Answer from the drawing. Dimensions are ordinates in mm from the lowest x, y and z of the part. Coordinates: 2 decimals unless noted, no trailing zeros. Order: outer loops, then holes, each group sorted by start corner. A loop starts at its lowest first (then second) coordinate and runs counter-clockwise, first axis right, second up. Notation, with made-up numbers: (-1, -30.75) - (33, -30.75) arc R12 cw to (33, -10.75) - close; hole circle Ø11 at (40.25, 14.25). An arc over 180 degrees is marked (long way). Answer as a JSON object with one key per item and string values. Group by question number.
1) Find the intervals of material crossed by line 1 along X through (y, z) = (47.5, 5); line 2 along X through (y, z) = (156, 6.5), in increasing order.
2) Section C-C (y = 167) is taken. Give the vertices of the cut face in (x, z).
3) Section B-B (x = 47.5) is taken. Give the vertices of the cut face in (y, z).
4) Section A-A (z = 3) is taken. Give the vertices of the cut face in (x, y).
5) Each of these flat-tipped pins is pushed along its axis until it touches: P1, Ø4, axis at y = 99.5, z = 1.5, coming from the -X side; P2, Ø5, axis at x = 9, z = 2.5, coming from the -Y side; P3, Ø1, axis at y = 130.5, z = 7, coming from the +X side; P4, Ø1, axis at y = 42.5, z = 3, coming from the +X side. Where does it stop, or does it pass through?
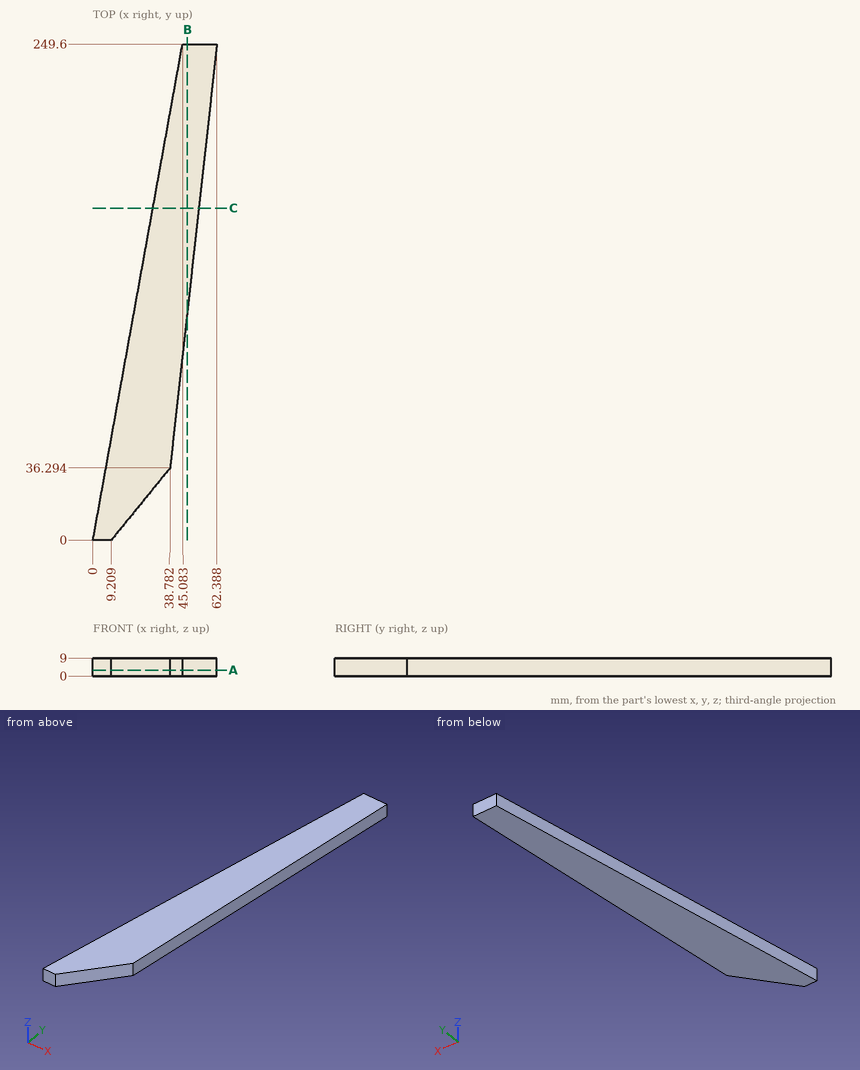
Report:
{
 "1": {"line 1": "x = 8.58 to 40.02", "line 2": "x = 28.18 to 52.03"},
 "2": {"outline": "(30.16, 0) - (53.25, 0) - (53.25, 9) - (30.16, 9) - close"},
 "3": {"outline": "(115.07, 0) - (249.6, 0) - (249.6, 9) - (115.07, 9) - close"},
 "4": {"outline": "(0, 0) - (9.21, 0) - (38.78, 36.29) - (62.39, 249.6) - (45.08, 249.6) - close"},
 "5": {"P1": "stops at x = 17.61", "P2": "stops at y = 0", "P3": "stops at x = 49.26", "P4": "stops at x = 39.52"}
}
